The listing builds one solid part. Answer for the finished solid, in the listing's coordinates (mm). A direction names the side the tool comes from. Coordinates: 2 decimals unless noted, no trailing zeros. Loops run counter-clockwise (first coordinate to the right, second up) from the corner with the lowest first, then second, coordinate; pieces in that order, holes last. Notation, with made-up numbers: M 1.5,20 L 46.5,20 A27 ccw 46.5,41 Z; hole C 49.25,63.25 d3. An arc over 180 degrees is marked long. Answer as a JSON object with one key per item and string values. Group by question number.
1. Straight lines are drawn through the part: L1, parallel to X at y = 15, z = 2; L2, parallel to Z at x = 47.5, y = 12.5; L3, parallel to Y at x = 25.5, z = 3.5. For each, find the intervals that lie inside material, in ascending order.
2. A cutting plane is placed at C-C on z = 46. Give the vertices of the cut face in (x, y), and give its area (3 significant figures).
3. A cutting plane is placed at A-A on y = 0. Give the vertices of the cut face in (x, z), and give its area (3 significant figures).
4. Determine the mould class of faces 1 (the face through (123.52, 0, 5)), 2 (the face through (114.524, 26.676, 34.65)), 3 (the face through (30, 52, 60)), 4 (the face through (22.507, -51.632, 34.65)) for opening direction X: released by +X, released by -X, zero draft, split by the parting line, or undercut.
5. Given pin 1 (4 mm diameter, centred on x = 114.4, y = 15.5, fed in from -Z); pin 2 (10 mm diameter, centred on x = 82.5, z = 17.5, fed in from +Y); pin 3 (6 mm diameter, centred on x = 83.4, y = -15.5, fed in from +Z); pin 4 (8 mm diameter, centred on y = -51.5, z = 32.5, fed in from +X), each flat-ended and moving along its own axis, determine where each tip first touches the part or whether it passes through.
6. A cutting plane is placed at B-B on z = 5. Give the vertices of the cut face in (x, y), and give its area (3 significant figures).
7. A cutting plane is placed at D-D on x = 98. Give the vertices of the cut face in (y, z).
8. For faces 5 (the face through (96, 31.5, 5)), 6 (the face through (85.784, -14.749, 4.93)), 7 (the face through (-67.493, 0.33, 34.65)), determine the directions among +Z, -Z, +X, -X, +Y, -Y from which every point of the face is accessible in a straight line to the end or side of a thin tool.
from build123d import *

# Parameters (mm, degrees)
F1_DEPTH = 10
F2_R     = 2.5
F3_DEPTH = 10
F2_R_2   = 11.5
F4_DEPTH = 10
F5_R     = 7.5
F5_R_2   = 4
F6_DEPTH = 50


with BuildPart() as f1:
    # F0 (on Top) → F1 (new body)
    with BuildSketch(Plane.XY):
        with BuildLine():
            ThreePointArc((68.064308, -31.5), (73.245556, -16.127258), (75, 0))
            ThreePointArc((75, 0), (73.245556, 16.127258), (68.064308, 31.5))
            ThreePointArc((68.064308, 31.5), (-75, 0), (68.064308, -31.5))
        make_face()
        with BuildLine():
            ThreePointArc((68.064308, 31.5), (73.245556, 16.127258), (75, 0))
            ThreePointArc((75, 0), (73.245556, -16.127258), (68.064308, -31.5))
            Line((68.064308, -31.5), (123.52035, -31.5))
            Line((123.52035, -31.5), (123.52035, 31.5))
            Line((123.52035, 31.5), (68.064308, 31.5))
        make_face()
    extrude(amount=F1_DEPTH)

    # F2 (on face) → F3 (cut, through all)
    with BuildSketch(Plane.XY):
        with Locations((114.399239, 15.5)):
            Circle(F2_R)
        with Locations((83.399239, 15.5)):
            Circle(F2_R)
        with Locations((83.399239, -15.5)):
            Circle(F2_R)
        with Locations((114.399239, -15.5)):
            Circle(F2_R)
    extrude(amount=F3_DEPTH, mode=Mode.SUBTRACT)

    # F2 (on face) → F4 (cut, through all)
    with BuildSketch(Plane.XY):
        with Locations((98.899239, 0)):
            Circle(F2_R_2)
    extrude(amount=F4_DEPTH, mode=Mode.SUBTRACT)

    # F5 (on face) → F6 (join)
    with BuildSketch(Plane.XY.offset(10)):
        with Locations((-60, 0)):
            Circle(F5_R)
        with Locations((30, 51.961524)):
            Circle(F5_R)
        with Locations((30, -51.961524)):
            Circle(F5_R)
        with Locations((75.972773, -26.5)):
            Circle(F5_R_2)
        with Locations((118.52035, -26.5)):
            Circle(F5_R_2)
        with Locations((75.264111, 26.5)):
            Circle(F5_R_2)
        with Locations((118.52035, 26.5)):
            Circle(F5_R_2)
    extrude(amount=F6_DEPTH)


solid = f1.part
From the geometry:
{
 "1": {"L1": "x = -73.48 to 80.95, 85.85 to 111.95, 116.85 to 123.52", "L2": "z = 0 to 10", "L3": "y = -70.53 to 70.53"},
 "2": {"outline": "C -60,0 d15; C 30,-51.96 d15; C 30,51.96 d15; C 75.26,26.5 d8; C 75.97,-26.5 d8; C 118.52,-26.5 d8; C 118.52,26.5 d8", "area": "731 mm²"},
 "3": {"outline": "M -75,0 L 87.4,0 L 87.4,10 L -52.5,10 L -52.5,60 L -67.5,60 L -67.5,10 L -75,10 Z; M 110.4,0 L 123.52,0 L 123.52,10 L 110.4,10 Z", "area": "2,510 mm²"},
 "4": {"face 1": "released by +X", "face 2": "undercut", "face 3": "zero draft", "face 4": "split by the parting line"},
 "5": {"pin 1": "passes through", "pin 2": "stops at y = 29.82", "pin 3": "stops at z = 10", "pin 4": "stops at x = 37.5"},
 "6": {"outline": "M 68.06,-31.5 L 123.52,-31.5 L 123.52,31.5 L 68.06,31.5 A75 ccw long Z; hole C 83.4,-15.5 d5; hole C 83.4,15.5 d5; hole C 98.9,0 d23; hole C 114.4,-15.5 d5; hole C 114.4,15.5 d5", "area": "20,400 mm²"},
 "7": {"outline": "M -31.5,0 L -11.46,0 L -11.46,10 L -31.5,10 Z; M 11.46,0 L 31.5,0 L 31.5,10 L 11.46,10 Z"},
 "8": {"face 5": "+Z, -Z, +X, +Y", "face 6": "+Z, -Z", "face 7": "+Z"}
}
